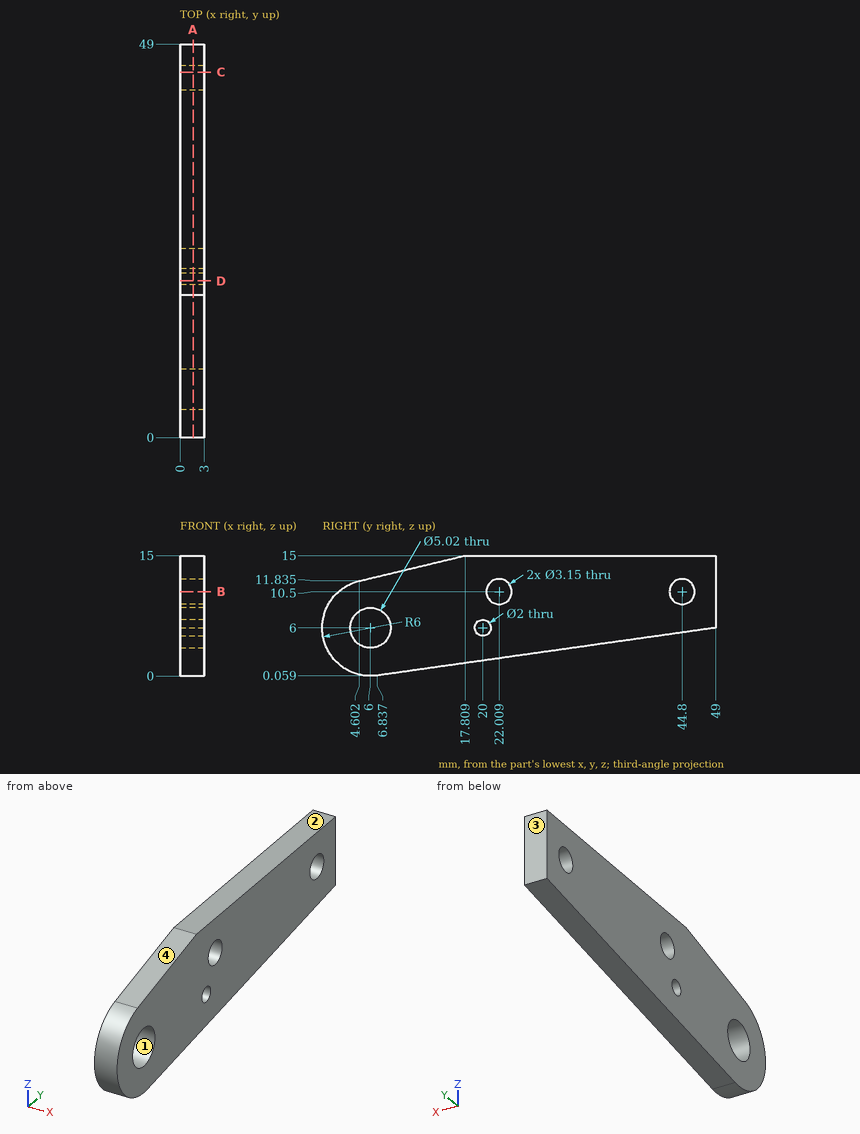
The figure shows three views and two pictorial views of one solid part (mm, origin at its lowest corner). Answer the questions. Round coordinates to 2 decimals unless told otherwise and drop trailing zeros. Loops run counter-clockwise (first coordinate to the right, second up) from the corner with the lowest first, then second, coordinate; pieces in that order, holes last. Notation, with made-up numbers: M 45,-37 L 55,-37 A27 ccw 55,-19 Z; hole C 64,81 d8. An arc over 180 degrees is marked long. Use CSV: the item, a comma, the result in double quotes.
Q1. Section A-A, the plane x = 1.6 is taken. State how many separate pieces and enclosed holes the cut face has, then the cut area to 3 significant figures.
Determined:
separate pieces,"1"
enclosed holes,"4"
area,"519 mm2"
Q2. Consider L1, parallel to Y at x = 0.65, z = 7.25 (1 decimal); L2, parallel to Z at x = 2.6, y = 6.5; L3, parallel to Z at x = 0.7, y = 7.5. Determine where each line is inside the solid, lowest interval first.
Determined:
L1,"0.1 to 3.8, 8.2 to 49"
L2,"0.02 to 3.54, 8.46 to 12.29"
L3,"0.15 to 3.99, 8.01 to 12.53"
Q3. Section D-D, the plane y = 19.5 is taken. Determine the outline of the cut face in (x, z).
Determined:
outline,"M 0,1.84 L 3,1.84 L 3,5.13 L 0,5.13 Z; M 0,6.87 L 3,6.87 L 3,15 L 0,15 Z"
Q4. Section B-B, the plane z = 10.5 is taken. Determine the outline of the cut face in (x, y) (1 decimal), then the cut area to 3 significant figures.
Determined:
outline,"M 0,2 L 3,2 L 3,20.4 L 0,20.4 Z; M 0,23.6 L 3,23.6 L 3,43.2 L 0,43.2 Z; M 0,46.4 L 3,46.4 L 3,49 L 0,49 Z"
area,"122 mm2"
Q5. The mould has two halves that part along Y. Classify the marked faces 1, 2, 3 and 4: pulls with the +Y half, pulls with the -Y half, needs draft (parallel to the pull), parting line crosses it, or undercut.
Determined:
face 1,"undercut"
face 2,"needs draft"
face 3,"pulls with the +Y half"
face 4,"pulls with the -Y half"
Q6. Section C-C, the plane y = 45.5 is taken. Determine the outline of the cut face in (x, z), then the cut area to 3 significant figures.
Determined:
outline,"M 0,5.51 L 3,5.51 L 3,9.09 L 0,9.09 Z; M 0,11.91 L 3,11.91 L 3,15 L 0,15 Z"
area,"20.0 mm2"
